Part model, mm, in its own coordinate system. Coordinates: 2 decimals unless noted, no trailing zeros. Write each loop counter-clockwise with the first axis right and the second up, starting at its lowest first coordinate (ties: lowest second). Pieces come first, ordered by that corner, then holes. Notation, with made-up numbers: (51, 81.25) - (110, 81.25) arc R27 cw to (110, 113.25) - close; hole circle Ø6 at (9.25, 54.25). An arc over 180 degrees is marked (long way). Use a Markdown table: item, result.
```python
from build123d import *

# Parameters (mm, degrees)
F0_R     = 1.5
F1_DEPTH = 2
F2_R     = 0.4


with BuildPart() as f1:
    # F0 (on Top) → F1 (new body)
    with BuildSketch(Plane.XY):
        with BuildLine():
            ThreePointArc((-3.72678, 3.333333), (-1.78411, -4.670862), (5, 0))
            ThreePointArc((5, 0), (4.670862, 1.78411), (3.72678, 3.333333))
            ThreePointArc((3.72678, 3.333333), (2.041241, 4.564355), (0, 5))
            ThreePointArc((0, 5), (-2.041241, 4.564355), (-3.72678, 3.333333))
        make_face()
        with BuildLine():
            ThreePointArc((0, 5), (2.041241, 4.564355), (3.72678, 3.333333))
            ThreePointArc((3.72678, 3.333333), (2.690663, 5.145215), (2.48452, 7.222222))
            ThreePointArc((2.48452, 7.222222), (1.666667, 5.63661), (0, 5))
        make_face()
        with BuildLine():
            ThreePointArc((-2.48452, 7.222222), (-2.690663, 5.145215), (-3.72678, 3.333333))
            ThreePointArc((-3.72678, 3.333333), (-2.041241, 4.564355), (0, 5))
            ThreePointArc((0, 5), (-1.666667, 5.63661), (-2.48452, 7.222222))
        make_face()
        with BuildLine():
            ThreePointArc((-2.48452, 7.222222), (-1.666667, 5.63661), (0, 5))
            ThreePointArc((0, 5), (1.666667, 5.63661), (2.48452, 7.222222))
            ThreePointArc((2.48452, 7.222222), (2.496127, 7.360896), (2.5, 7.5))
            ThreePointArc((2.5, 7.5), (-0.139104, 9.996127), (-2.48452, 7.222222))
        make_face()
        with Locations((0, 7.5)):
            Circle(F0_R, mode=Mode.SUBTRACT)
    extrude(amount=F1_DEPTH)

    # F2
    f2_edges = [f1.edges().sort_by_distance(p)[0] for p in [
        (4.670862, 1.78411, 0),
        (2.690663, 5.145215, 0),
        (0, 10, 0),
        (-2.690663, 5.145215, 0),
        (-1.78411, -4.670862, 0),
        (-1.5, 7.5, 0),
        (-1.78411, -4.670862, 2),
        (4.670862, 1.78411, 2),
        (2.690663, 5.145215, 2),
        (0, 10, 2),
        (-2.690663, 5.145215, 2),
        (-1.5, 7.5, 2),
    ]]
    fillet(f2_edges, radius=F2_R)


solid = f1.part
```
Item 1: Drop a flat-ended pin along its axis: P1, Ø1, axis at y = 3, z = 0, coming from the +X side. Give the stop position or say it passes through.
From the geometry:
| item | result |
|---|---|
| P1 | x = 4.26 |
Item 2: Band-saw the part on A-A, the plane z = 1.8. Give the cut face in (x, y), then the cut area to 3 significant figures.
From the geometry:
| item | result |
|---|---|
| outline | (-3.69, 3.3) arc R4.95 ccw (long way) to (4.95, 0) arc R4.95 ccw to (3.69, 3.3) arc R5.05 cw to (2.43, 7.23) arc R2.45 ccw to (2.45, 7.5) arc R2.45 ccw (long way) to (-2.43, 7.23) arc R5.05 cw to start; hole circle Ø3.11 at (0, 7.5) |
| area | 93.2 mm^2 |
Item 3: Two-plate mould, pull along X, no slides. Class faces 1 (the face through (0, 10, 1)), 2 (the face through (0, 1, 0)), 3 (the face through (0, 6, 1)): pulls with the +X half, pulls with the -X half, needs draft (parallel to the pull), parting line crosses it, or undercut.
From the geometry:
| item | result |
|---|---|
| face 1 | parting line crosses it |
| face 2 | needs draft |
| face 3 | undercut |
Item 4: Drill centre lines: probe 1 along Y at (x, z) = (0, 1.3); probe 2 along Y at (x, z) = (-1, 1.7); probe 3 along X at (y, z) = (8, 0.7). Where is each one in solid material? Low to high.
From the geometry:
| item | result |
|---|---|
| probe 1 | -5 to 6, 9 to 10 |
| probe 2 | -4.89 to 6.36, 8.64 to 9.78 |
| probe 3 | -2.45 to -1.41, 1.41 to 2.45 |
Item 5: Band-saw the part on B-B, the plane z = 1.1. Give the cut face in (x, y).
From the geometry:
| item | result |
|---|---|
| outline | (-3.73, 3.33) arc R5 ccw (long way) to (5, 0) arc R5 ccw to (3.73, 3.33) arc R5 cw to (2.48, 7.22) arc R2.5 ccw to (2.5, 7.5) arc R2.5 ccw (long way) to (-2.48, 7.22) arc R5 cw to start; hole circle Ø3 at (0, 7.5) |
